The model under review builds one solid part; all positions refer to its coordinate system, in mm. Face numbers are marked on the shaded views. A direction names the side the tool comes from. Round coordinates to 2 decimals unless told otherwise and drop trailing zeros. Write each loop counter-clockwise with the first axis right and the second up, starting at its lowest first coordinate (ties: lowest second). Pieces come first, ordered by that corner, then holes. Notation, with made-up numbers: (58, -35.75) -> (98, -35.75) arc R28 ccw to (98, 0.25) -> close; hole circle Ø10 at (-32, 44.25). An arc over 180 degrees is marked (long way). Use CSV: the item, a comma, the result in double quotes. Start each with the question number.
1) For pin 1 Ø1 at (x, z) = (89.5, -18) entering from -Y, flat-tipped, find the tip position at first contact; note if it passes through.
2) Mouldability with a two-part tool opening along Z and no side actions: class the marked faces 3, 4 and 5 as released by +Z, released by -Z, zero draft, split by the parting line, or undercut.
3) Take a section at A-A, the plane x = 85. Give the boundary of the cut face in (y, z).
4) Take a section at C-C, the plane x = 0. Give the boundary of the cut face in (y, z).
5) Machinability: for the marked faces 1 and 2, which of the approach directions +Z, -Z, +X, -X, +Y, -Y give a long, thin tool a straight path to every point of the face, cutting with its end or side? Answer none if there is none.
6) Take a section at B-B, the plane z = 0. Give the boundary of the cut face in (x, y).
7) Wall thickness on probe 1 along Z at (x, y) = (0, -72); probe 2 along Z at (x, y) = (-85, -71); probe 3 along Y at (x, z) = (97, 9): over which ranges is each line inside the solid? List them lowest first. Write a range as [from, to].
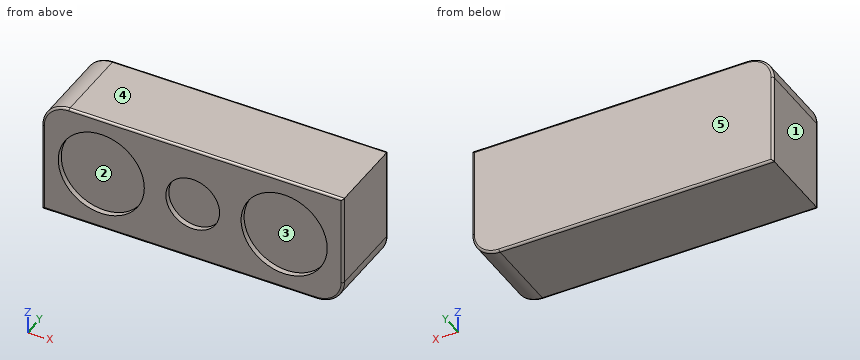
from build123d import *

# Parameters (mm, degrees)
F1_DEPTH = 75
F2_R     = 2
F3_R     = 25
F3_R_2   = 40
F4_DEPTH = 5


with BuildPart() as f1:
    # F0 (on Front) → F1 (new body)
    with BuildSketch(Plane.XZ):
        with BuildLine():
            Line((-140, 30), (-140, -55))
            Line((-140, -55), (115, -55))
            ThreePointArc((115, -55), (132.6776695297, -47.6776695297), (140, -30))
            Line((140, -30), (140, 55))
            Line((140, 55), (-115, 55))
            ThreePointArc((-115, 55), (-132.6776695297, 47.6776695297), (-140, 30))
        make_face()
    extrude(amount=F1_DEPTH)

    # F2
    f2_edges = [f1.edges().sort_by_distance(p)[0] for p in [
        (-132.67767, -75, 47.67767),
        (-140, -75, -12.5),
        (-12.5, -75, -55),
        (132.67767, -75, -47.67767),
        (140, -75, 12.5),
        (12.5, -75, 55),
        (-132.67767, 0, 47.67767),
        (-140, 0, -12.5),
        (-12.5, 0, -55),
        (132.67767, 0, -47.67767),
        (140, 0, 12.5),
        (12.5, 0, 55),
    ]]
    fillet(f2_edges, radius=F2_R)

    # F3 (on face) → F4 (cut)
    with BuildSketch(Plane.XZ.offset(75)):
        Circle(F3_R)
        with Locations((-85, 0)):
            Circle(F3_R_2)
        with Locations((85, 0)):
            Circle(F3_R_2)
    extrude(amount=-F4_DEPTH, mode=Mode.SUBTRACT)


solid = f1.part
Values found:
1,pin 1,"y = -70"
2,face 3,"undercut"
2,face 4,"released by +Z"
2,face 5,"zero draft"
3,outline,"(-75, -53) arc R2 ccw to (-73, -55) -> (-2, -55) arc R2 ccw to (0, -53) -> (0, 53) arc R2 ccw to (-2, 55) -> (-73, 55) arc R2 ccw to (-75, 53) -> (-75, 40) -> (-70, 40) -> (-70, -40) -> (-75, -40) -> close"
4,outline,"(-75, -53) arc R2 ccw to (-73, -55) -> (-2, -55) arc R2 ccw to (0, -53) -> (0, 53) arc R2 ccw to (-2, 55) -> (-73, 55) arc R2 ccw to (-75, 53) -> (-75, 25) -> (-70, 25) -> (-70, -25) -> (-75, -25) -> close"
5,face 1,"+Z, -Z, -X, +Y, -Y"
5,face 2,"-Y"
6,outline,"(-140, -73) arc R2 ccw to (-138, -75) -> (-125, -75) -> (-125, -70) -> (-45, -70) -> (-45, -75) -> (-25, -75) -> (-25, -70) -> (25, -70) -> (25, -75) -> (45, -75) -> (45, -70) -> (125, -70) -> (125, -75) -> (138, -75) arc R2 ccw to (140, -73) -> (140, -2) arc R2 ccw to (138, 0) -> (-138, 0) arc R2 ccw to (-140, -2) -> close"
7,probe 1,"[-55, -25], [25, 55]"
7,probe 2,"[-55, -40], [40, 55]"
7,probe 3,"[-70, 0]"
